```python
from build123d import *

# Parameters (mm, degrees)
SKETCH_1_W          = 30
SKETCH_1_H          = 20
EXTRUDE_1_DEPTH     = 4.2
SKETCH_2_R          = 4.15
CUT_EXTRUDE_1_DEPTH = 19.510537539
SKETCH_3_W          = 8
SKETCH_3_H          = 8.5
CUT_EXTRUDE_2_DEPTH = 19.510537539
EXTRUDE_2_DEPTH     = 2
SKETCH_5_R          = 2.25
CUT_EXTRUDE_3_DEPTH = 19.510537539
SKETCH_6_W          = 8
SKETCH_6_H          = 2
CUT_EXTRUDE_4_DEPTH = 20.064102392
SKETCH_7_R          = 1.1
CUT_EXTRUDE_5_DEPTH = 20.064102392
SKETCH_8_W          = 2.8
SKETCH_8_H          = 2.8
EXTRUDE_3_DEPTH     = 3


with BuildPart() as part:
    # 草图1 → 凸台-拉伸1 (new body)
    with BuildSketch(Plane(origin=(0, 0, 0), x_dir=(1, 0, 0), z_dir=(0, 1, 0))):
        Rectangle(SKETCH_1_W, SKETCH_1_H)
    extrude(amount=EXTRUDE_1_DEPTH)

    # 草图2 → 切除-拉伸1 (cut, through all)
    with BuildSketch(Plane(origin=(0, 4.2, 0), x_dir=(1, 0, 0), z_dir=(0, 1, 0))):
        with Locations(Location((-7.5, 3, 0), (0, 0, 270))):
            Circle(SKETCH_2_R)
        with Locations(Location((7.5, 3, 0), (0, 0, 270))):
            Circle(SKETCH_2_R)
    extrude(amount=-CUT_EXTRUDE_1_DEPTH, mode=Mode.SUBTRACT)

    # 草图3 → 切除-拉伸2 (cut, through all)
    with BuildSketch(Plane(origin=(0, 4.2, 0), x_dir=(1, 0, 0), z_dir=(0, 1, 0))):
        with Locations((0, -5.75)):
            Rectangle(SKETCH_3_W, SKETCH_3_H)
    extrude(amount=-CUT_EXTRUDE_2_DEPTH, mode=Mode.SUBTRACT)

    # 草图4 → 凸台-拉伸2 (add)
    with BuildSketch(Plane(origin=(0, 4.2, 0), x_dir=(1, 0, 0), z_dir=(0, 1, 0))):
        Polygon((-4, -1.5), (4, -1.5), (4, -10), (15, -10), (15, 10), (-15, 10), (-15, -10), (-4, -10), align=None)
    extrude(amount=EXTRUDE_2_DEPTH)

    # 草图5 → 切除-拉伸3 (cut, through all)
    with BuildSketch(Plane.XZ.offset(-4.2)):
        with Locations(Location((-7.5, -3, 0), (0, 0, 270))):
            Circle(SKETCH_5_R)
        with Locations(Location((7.5, -3, 0), (0, 0, 270))):
            Circle(SKETCH_5_R)
    extrude(amount=-CUT_EXTRUDE_3_DEPTH, mode=Mode.SUBTRACT)

    # 草图6 → 切除-拉伸4 (cut, through all)
    with BuildSketch(Plane(origin=(0, 6.2, 0), x_dir=(1, 0, 0), z_dir=(0, 1, 0))):
        with Locations((0, 9)):
            Rectangle(SKETCH_6_W, SKETCH_6_H)
    extrude(amount=-CUT_EXTRUDE_4_DEPTH, mode=Mode.SUBTRACT)

    # 草图7 → 切除-拉伸5 (cut, through all)
    with BuildSketch(Plane(origin=(0, 6.2, 0), x_dir=(1, 0, 0), z_dir=(0, 1, 0))):
        with Locations(Location((-7, -6, 0), (0, 0, 270))):
            Circle(SKETCH_7_R)
        with Locations(Location((7, -6, 0), (0, 0, 90))):
            Circle(SKETCH_7_R)
    extrude(amount=-CUT_EXTRUDE_5_DEPTH, mode=Mode.SUBTRACT)

    # 草图8 → 凸台-拉伸3 (add)
    with BuildSketch(Plane.XZ):
        with Locations((0, -5)):
            Rectangle(SKETCH_8_W, SKETCH_8_H)
    extrude(amount=EXTRUDE_3_DEPTH)


solid = part.part
```
Can you work these out from the model? Positions are in its coordinate system, mm. A direction names the side the tool comes from. Coordinates: 2 decimals unless noted, no trailing zeros. Loops run counter-clockwise (first coordinate to the right, second up) from the corner with the lowest first, then second, coordinate; pieces in that order, holes last. Notation, with made-up numbers: (12, 61.25) - (22, 61.25) arc R10 cw to (22, 72.25) - close; hole circle Ø4 at (-2.5, 71.25). An arc over 180 degrees is marked (long way). Use a Markdown table: item, result.
Item 1: For faces 1 (the face through (1.4, -1, -5)), 2 (the face through (-4, 2.13, -0.77)), 3 (the face through (0, 3, -8)), 4 (the face through (-4, 3, 6)), 5 (the face through (0, -1, -3.6)), which set-ups out of +Z, -Z, +X, -X, +Y, -Y let a thin tool reach every point of the face, with its end or its side?
Numbers:
| item | result |
|---|---|
| face 1 | +Z, -Z, +X, -Y |
| face 2 | -Y |
| face 3 | -Z, +Y, -Y |
| face 4 | +Z, +Y, -Y |
| face 5 | +Z, +X, -X, -Y |
Item 2: I want a section at B-B on y = 4.75. Please give me the cut outline in (x, z).
Numbers:
| item | result |
|---|---|
| outline | (-15, -10) - (-4, -10) - (-4, -8) - (4, -8) - (4, -10) - (15, -10) - (15, 10) - (4, 10) - (4, 1.5) - (-4, 1.5) - (-4, 10) - (-15, 10) - close; hole circle Ø4.5 at (-7.5, -3); hole circle Ø2.2 at (-7, 6); hole circle Ø4.5 at (7.5, -3); hole circle Ø2.2 at (7, 6) |
Item 3: If I drill on probe 1 along X at (y, z) = (2.2, -3); probe 2 along X at (y, z) = (5.6, -3); probe 3 along X at (y, z) = (3.75, 6), over which ranges is the centre line in solid material (lowest first)? Write a range as from..to.
Numbers:
| item | result |
|---|---|
| probe 1 | x = -15..-11.65, -3.35..3.35, 11.65..15 |
| probe 2 | x = -15..-9.75, -5.25..5.25, 9.75..15 |
| probe 3 | x = -15..-8.1, -5.9..-4, 4..5.9, 8.1..15 |
Item 4: Will these pins go through, and if not, where does the flat tip stop? pin 1 (1.4 mm diameter, centred on x = 0.5, y = -1, fed in from +Z); pin 2 (1.4 mm diameter, centred on y = -1.5, z = -5, fed in from +X); pin 3 (2.5 mm diameter, centred on x = 7, z = -4, fed in from -Y).
Numbers:
| item | result |
|---|---|
| pin 1 | stops at z = -3.6 |
| pin 2 | stops at x = 1.4 |
| pin 3 | stops at y = 4.2 |
Item 5: I want a section at D-D on x = -1. Please give me the cut outline in (y, z).
Numbers:
| item | result |
|---|---|
| outline | (-3, -6.4) - (0, -6.4) - (0, -8) - (6.2, -8) - (6.2, 1.5) - (0, 1.5) - (0, -3.6) - (-3, -3.6) - close |
Item 6: We'd pull the mould along Z, two halves only. Please class faces 6 (the face through (9, 3, 10)), 7 (the face through (10, 3, -10)), 8 (the face through (11.615, 2.129, -3.54)), 9 (the face through (-4, 3, -9)): released by +Z, released by -Z, zero draft, split by the parting line, or undercut.
Numbers:
| item | result |
|---|---|
| face 6 | released by +Z |
| face 7 | released by -Z |
| face 8 | undercut |
| face 9 | zero draft |
Item 7: I want a section at C-C on z = -3. Please give me the cut outline in (x, y), and give its area (3 significant figures).
Numbers:
| item | result |
|---|---|
| outline | (-15, 0) - (-11.65, 0) - (-11.65, 4.2) - (-9.75, 4.2) - (-9.75, 6.2) - (-15, 6.2) - close; (-5.25, 4.2) - (-3.35, 4.2) - (-3.35, 0) - (3.35, 0) - (3.35, 4.2) - (5.25, 4.2) - (5.25, 6.2) - (-5.25, 6.2) - close; (9.75, 4.2) - (11.65, 4.2) - (11.65, 0) - (15, 0) - (15, 6.2) - (9.75, 6.2) - close |
| area | 98.3 mm2 |
Item 8: I want a section at A-A on z = 4.5. Please give me the cut outline in (x, y).
Numbers:
| item | result |
|---|---|
| outline | (-15, 0) - (-4, 0) - (-4, 6.2) - (-15, 6.2) - close; (4, 0) - (15, 0) - (15, 6.2) - (4, 6.2) - close |
